Could you check a few things on this model? Use its own coordinates, in mm. Face numbers are marked on the shaded views. A direction names the side the tool comes from. Coordinates: 2 decimals unless noted, no trailing zeros. Write each loop counter-clockwise with the first axis right and the second up, starting at its lowest first coordinate (ties: lowest second). Pieces come first, ordered by that corner, then holes. Notation, with made-up numbers: (20, -33) - (65, -33) arc R17 ccw to (65, -13) - close; hole circle Ø11 at (48, 74.5). An arc over 180 degrees is marked (long way). Write item = value, one per line. Start each with the question number.
```python
from build123d import *

# Parameters (mm, degrees)
F4_COPIES_COUNT = 4
F6_DEPTH        = 7


# Not quite as in the source:
# - a pattern or mirror of a feature is missing from the dataset's text; its kind, count and spacing are read off the source's solid


with BuildPart() as f1:
    # F0 (on Front) → F1 (revolve)
    with BuildSketch(Plane.XZ):
        Polygon((12.65, -40), (25.25, -40), (25.25, -35), (28.1, -35), (28.1, -19.5), (20.4, -19.5), (20.4, -13.25), (18.4, -13.25), (13.9, -37), (12.65, -37), align=None)
    revolve(axis=Axis((0, 0, -3.8875962891), (0, 0, -1)))

    # F3 (on Front) → F4 (revolve, cut)
    with BuildSketch(Plane.XZ):
        Polygon((27.7907, -19.5), (25.9972140193, -19.5), (25.9972140193, -22.421), (27.5621, -22.421), align=None)
    f4 = revolve(axis=Axis((25.9972140193, 0, -20.9605), (0, 0, 1)), mode=Mode.SUBTRACT)

    # F4_copies: F4 ×4 about axis
    f4_copies_axis = Axis((0, 0, 0), (0, 0, 1))
    for i in range(1, F4_COPIES_COUNT):
        add(f4.rotate(f4_copies_axis, i * 360 / F4_COPIES_COUNT), mode=Mode.SUBTRACT)

    # F5 (on face) → F6 (cut)
    with BuildSketch(Plane(origin=(0, 0, -40), x_dir=(1, 0, 0), z_dir=(0, 0, -1))):
        with BuildLine():
            Line((-3.5, 18.75), (-3.5, 15.15))
            Line((-3.5, 15.15), (3.5, 15.15))
            Line((3.5, 15.15), (3.5, 18.75))
            ThreePointArc((3.5, 18.75), (2.4748737342, 21.2248737342), (0, 22.25))
            ThreePointArc((0, 22.25), (-2.4748737342, 21.2248737342), (-3.5, 18.75))
        make_face()
        with BuildLine():
            ThreePointArc((23.25, 3), (22.6642135624, 4.4142135624), (21.25, 5))
            Line((21.25, 5), (16.15, 5))
            Line((16.15, 5), (16.15, -5))
            Line((16.15, -5), (21.25, -5))
            ThreePointArc((21.25, -5), (22.6642135624, -4.4142135624), (23.25, -3))
            Line((23.25, -3), (23.25, 3))
        make_face()
    extrude(amount=-F6_DEPTH, mode=Mode.SUBTRACT)


solid = f1.part
```
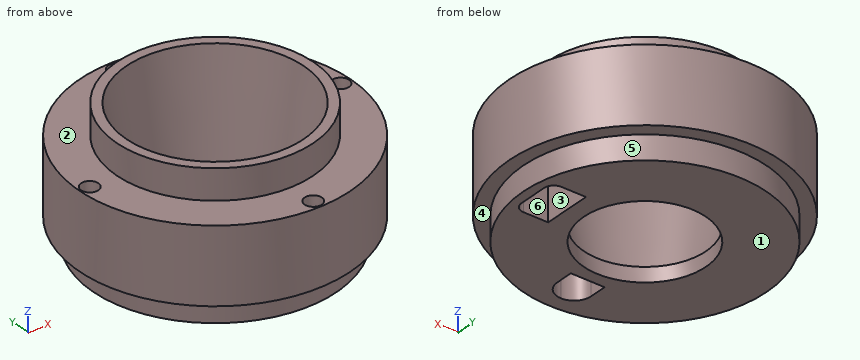
1) Suppose I cut it at C-C on x = 19.5. Please give me the cut outline in (y, z).
2) Which directions (+Z, -Z, +X, -X, +Y, -Y) give clear straight access to the entire face, cutting with the end or side of a thin tool? Please do the marked faces 1, 2 and 3.
3) Suppose I cut it at B-B on z = -28. Please give me the cut outline in (x, y).
4) For P1, Ø2, axis at y = -1, z = -35.5, coming from the +X side; P2, Ø3.5, axis at x = 0.5, y = 25.5, coming from the +Z side; P3, Ø2, axis at x = 1, z = -20.5, coming from the -Y side; P4, Ø23, axis at x = 0, y = 0, coming from the +Z side, each with a flat end and sliding along its axis, tell me the tip position at first contact or that it passes through.
5) If I drill on probe 1 along X at (y, z) = (0, -38.6); probe 2 along Y at (x, z) = (0, -38.8); probe 3 along X at (y, z) = (1.5, -36.5), over which ranges is the centre line in solid material (lowest first)? Write a range as [from, to].
6) Suppose I cut it at D-D on z = -20.75. Please give me the cut outline in (x, y), plus the area to 3 significant figures.
7) Thinking about a two-plate mould opening in X: for the marked faces 4, 5 and 6, which applies, +X half, -X half, draft (parallel to the pull), parting line (faces both ways), or undercut?
Reply:
q1.outline = (-20.23, -35) - (-16.04, -35) - (-16.04, -40) - (-5, -40) - (-5, -33) - (5, -33) - (5, -40) - (16.04, -40) - (16.04, -35) - (20.23, -35) - (20.23, -19.5) - (5.99, -19.5) - (5.99, -13.25) - (-5.99, -13.25) - (-5.99, -19.5) - (-20.23, -19.5) - close
q2.face_1 = -Z, +X, -X, +Y, -Y
q2.face_2 = +Z
q2.face_3 = -Z
q3.outline = circle Ø56.2 at (0, 0); hole circle Ø31.21 at (0, 0)
q4.P1 = 28.1
q4.P2 = -19.5
q4.P3 = -28.1
q4.P4 = through
q5.probe_1 = [-25.25, -12.65], [12.65, 16.15], [23.25, 25.25]
q5.probe_2 = [-25.25, -22.25], [-15.15, -12.65], [12.65, 25.25]
q5.probe_3 = [-25.21, -13.91], [13.91, 16.15], [23.25, 25.21]
q6.outline = circle Ø56.2 at (0, 0); hole circle Ø3.39 at (-26, 0); hole circle Ø33.96 at (0, 0); hole circle Ø3.39 at (0, -26); hole circle Ø3.39 at (0, 26); hole circle Ø3.39 at (26, 0)
q6.area = 1,540 mm^2
q7.face_4 = draft
q7.face_5 = parting line
q7.face_6 = undercut
